from build123d import *

# Parameters (mm, degrees)
SKETCH_1_R               = 9
SKETCH_1_R_2             = 6.25
EXTRUDE_1_DEPTH          = 200
SKETCH_2_R               = 1.75
CUT_EXTRUDE_1_DEPTH      = 10
CUT_EXTRUDE_1_DEPTH_BACK = 10


with BuildPart() as part:
    # ｽｹｯﾁ1 → ﾎﾞｽ - 押し出し1 (new body)
    with BuildSketch(Plane.XY):
        Circle(SKETCH_1_R)
        Circle(SKETCH_1_R_2, mode=Mode.SUBTRACT)
    extrude(amount=EXTRUDE_1_DEPTH)

    # ｽｹｯﾁ2 → ｶｯﾄ - 押し出し1 (cut, two sides)
    with BuildSketch(Plane(origin=(0, 0, 0), x_dir=(0, 0, -1), z_dir=(1, 0, 0))) as cut_extrude_1_sk:
        with Locations((-7.5, 0)):
            Circle(SKETCH_2_R)
        with Locations((-192.5, 0)):
            Circle(SKETCH_2_R)
        with Locations((-80, 0)):
            Circle(SKETCH_2_R)
        with Locations((-120, 0)):
            Circle(SKETCH_2_R)
        with Locations((-17.5, 0)):
            Circle(SKETCH_2_R)
        with Locations((-182.5, 0)):
            Circle(SKETCH_2_R)
    extrude(amount=CUT_EXTRUDE_1_DEPTH, mode=Mode.SUBTRACT)
    extrude(cut_extrude_1_sk.sketch, amount=-CUT_EXTRUDE_1_DEPTH_BACK, mode=Mode.SUBTRACT)


solid = part.part
CAD build for the part. Positions are in the model's coordinates, mm. Round coordinates to 2 decimals unless told otherwise and drop trailing zeros. Order: outer loops, then holes, each group sorted by start corner. A loop starts at its lowest first (then second) coordinate and runs counter-clockwise, first axis right, second up. Notation, with made-up numbers: M -9,11 L 38,11 A20 cw 38,29 Z; hole C 82,-14.5 d10. An arc over 180 degrees is marked long. Use one line per item in the form item = value.
Q1. Saw through at D-D on z = 135. Give the cut face in (x, y), then the cut area to 3 significant figures.
Recorded:
outline = C 0,0 d18; hole C 0,0 d12.5
area = 132 mm^2
Q2. Saw through at B-B on z = 80. Give the cut face in (x, y).
Recorded:
outline = M -8.83,-1.75 A9 ccw 8.83,-1.75 L 6,-1.75 A6.25 cw -6,-1.75 Z; M -8.83,1.75 L -6,1.75 A6.25 cw 6,1.75 L 8.83,1.75 A9 ccw Z
Q3. Saw through at C-C on y = 0. State how many separate pieces and enclosed holes the cut face has, then the cut area to 4 significant figures.
Recorded:
separate_pieces = 14
enclosed_holes = 0
area = 984.5 mm^2
Q4. Flat gauge pins, fed straight in: P1, Ø2, axis at x = -2.5, z = 164.5, coming from the +Y side; P2, Ø2, axis at y = 0, z = 120, coming from the -X side; P3, Ø3, axis at x = -3.5, z = 36.5, coming from the +Y side; P4, Ø1, axis at x = 6, z = 156, coming from the -Y side. Where does each tip first touch, or does it go through?
Recorded:
P1 = 8.87
P2 = through
P3 = 8.77
P4 = -7.12
Q5. Two-plate mould, pull along Y, no slides. Class faces 1 (the cylindrical face through (-7.479, 1.735, 182.728)), 2 (the cylindrical face through (8.584, 2.703, 98.6)), 3 (the flat face through (-6.13, -1.87, 200)): +Y half, -Y half, draft (parallel to the pull), parting line (faces both ways), or undercut.
Recorded:
face_1 = undercut
face_2 = parting line
face_3 = draft
Q6. Probe L1, parallel to Y at x = 0, z = 12; L2, parallel to X at y = 1.5, z = 132.5; L3, parallel to X at y = 4.25, z = 92.5. List the from-to ranges inside material, lowest first.
Recorded:
L1 = -9 to -6.25, 6.25 to 9
L2 = -8.87 to -6.07, 6.07 to 8.87
L3 = -7.93 to -4.58, 4.58 to 7.93
Q7. Saw through at A-A on x = 0. Give the cut face in (y, z), then the cut area to 3 significant figures.
Recorded:
outline = M -9,0 L -6.25,0 L -6.25,200 L -9,200 Z; M 6.25,0 L 9,0 L 9,200 L 6.25,200 Z
area = 1,100 mm^2
